Geometry: final body of the model. Coordinates: model frame, mm. A direction names the side the tool comes from. Coordinates: 2 decimals unless noted, no trailing zeros. Order: outer loops, then holes, each group sorted by start corner. A loop starts at its lowest first (then second) coordinate and runs counter-clockwise, first axis right, second up. Notation, with made-up numbers: M 64.5,32 L 94.5,32 A22 cw 94.5,41 Z; hole C -24.5,59 d2. An arc over 180 degrees is marked long. Write item = value, one per line. Start each with the question number.
```python
from build123d import *

# Parameters (mm, degrees)
F0_R     = 63.5
F1_DEPTH = 25.4
F2_W     = 63.917932
F2_H     = 72.142676
F3_DEPTH = 12.7


with BuildPart() as f1:
    # F0 (on Top) → F1 (new body)
    with BuildSketch(Plane.XY):
        Circle(F0_R)
    extrude(amount=F1_DEPTH)

    # F2 (on Right) → F3 (join, symmetric)
    with BuildSketch(Plane.YZ):
        with Locations((64.152928, 36.071338)):
            Rectangle(F2_W, F2_H)
    extrude(amount=F3_DEPTH, both=True)


solid = f1.part
```
Item 1: Section query C-C on z = 45. Output: boundary loops of the cut face in (x, y).
Item 2: Section query A-A on x = 0. Output: boundary loops of the cut face in (y, z), and give its area (3 significant figures).
Item 3: Section query D-D on y = 0. Output: boundary loops of the cut face in (x, z), and give its area (3 significant figures).
Item 4: First-contact query: pin 1 (5 mm diameter, centred on y = 55.5, z = 58, fed in from -X); pin 2 (6 mm diameter, centred on y = 37.5, z = 33.5, fed in from +X); pin 3 (12.5 mm diameter, centred on x = -6.5, z = 42.5, fed in from -Y). Flat tips, straight axial feed; report the tip coordinate or a pass-through.
Item 5: Reachability of faces 1 (the flat face through (-12.7, 64, 45)), 2 (the flat face through (0, 32.194, 48)), 3 (the cylindrical face through (-2.613, -63.446, 12.522)), 4 (the flat face through (-1, 0, 0)), 5 (the flat face through (12.7, 64, 45)) from +Z, -Z, +X, -X, +Y, -Y: full face, straight path, thin tool, end or side. Return the list, or none.
Item 6: Material intervals for probe 1 along Z at (x, y) = (38, -18); probe 2 along X at (y, z) = (56.5, 44.5); probe 3 along Y at (x, z) = (-10, 66.5), sorted ascending. Write a range as [from, to].
Item 7: Section query B-B on y = 35.5. Output: boundary loops of the cut face in (x, z).
Ans:
q1.outline = M -12.7,32.19 L 12.7,32.19 L 12.7,96.11 L -12.7,96.11 Z
q2.outline = M -63.5,0 L 96.11,0 L 96.11,72.14 L 32.19,72.14 L 32.19,25.4 L -63.5,25.4 Z
q2.area = 7,040 mm^2
q3.outline = M -63.5,0 L 63.5,0 L 63.5,25.4 L -63.5,25.4 Z
q3.area = 3,230 mm^2
q4.pin_1 = -12.7
q4.pin_2 = 12.7
q4.pin_3 = 32.19
q5.face_1 = +Z, -X, +Y
q5.face_2 = +Z, +X, -X, -Y
q5.face_3 = +Z, -Z
q5.face_4 = -Z, +X, -X, +Y, -Y
q5.face_5 = +Z, +X, +Y
q6.probe_1 = [0, 25.4]
q6.probe_2 = [-12.7, 12.7]
q6.probe_3 = [32.19, 96.11]
q7.outline = M -52.65,0 L 52.65,0 L 52.65,25.4 L 12.7,25.4 L 12.7,72.14 L -12.7,72.14 L -12.7,25.4 L -52.65,25.4 Z
